Solid Edge part; units mm, degrees
sketch "Sketch1" plane through (0, 0, 0) normal (0, -1, 0) x (1, 0, 0)
  circle A0 centre (0, 0) radius 6
extrude "Protrusion1" add sketch "Sketch1" along normal blind 3.6
sketch "Sketch2" plane through (0, -3.6, 0) normal (0, -1, 0) x (1, 0, 0)
  circle A0 centre (0, 0) radius 3
extrude "Protrusion2" add sketch "Sketch2" along normal blind 20
sketch "Sketch3" plane through (0, 0, 0) normal (0, 1, 0) x (0, 0, -1)
  line L0 (2.5, -1.4434) -> (2.5, 1.4434)
  line L1 (2.5, 1.4434) -> (0, 2.8868)
  line L2 (0, 2.8868) -> (-2.5, 1.4434)
  line L3 (-2.5, 1.4434) -> (-2.5, -1.4434)
  line L4 (-2.5, -1.4434) -> (0, -2.8868)
  line L5 (0, -2.8868) -> (2.5, -1.4434)
extrude "ExtrudedCutout_4" cut sketch "Sketch3" against normal blind 3
properties material "Nylon, general purpose"
Read the model definition and answer for the solid it produces. Units are mm, in the model's axes. A direction names the side the tool comes from. Round coordinates to 2 decimals unless told otherwise and drop trailing zeros. Write each loop counter-clockwise with the first axis right and the second up, starting at its lowest first coordinate (ties: lowest second). Pieces come first, ordered by that corner, then holes. Notation, with made-up numbers: M 57,-17.75 L 79,-17.75 A20 ccw 79,-3.75 Z; hole C -20,15 d3. An arc over 180 degrees is marked long. One line per item, written item: value.
Q1. Straight lines are drawn through the part: line 1 (Y direction, x = 4, z = 3.75); line 2 (Y direction, x = 0, z = -2.25); line 3 (Z direction, x = -1, y = -1). For each, find the intervals that lie inside material, in ascending order. Write a range as [from, to].
Data:
line 1: [-3.6, 0]
line 2: [-23.6, -3]
line 3: [-5.92, -2.5], [2.5, 5.92]
Q2. Which of the six approach directions +Z, -Z, +X, -X, +Y, -Y give full straight-line access (tool end or side, diameter ignored) to faces 5 (the flat face through (-1, -3.6, 3)), 6 (the flat face through (-2.175, -1.479, 1.233)), 7 (the flat face through (0, -23.6, 0))?
Data:
face 5: -Y
face 6: +Y
face 7: +Z, -Z, +X, -X, -Y
Q3. Find section D-D on x = -3.5. Write down the section's boundary in (y, z).
Data:
outline: M -3.6,-4.87 L 0,-4.87 L 0,4.87 L -3.6,4.87 Z
Q4. For a pull along Z with two mould halves and no side action, classify faces 1 (the flat face through (0, 0, -3)), 2 (the flat face through (0, -1, -2.5)), 3 (the cylindrical face through (-3, -13, 0)), 4 (the flat face through (2.155, -1.479, 1.267)) as +Z half, -Z half, draft (parallel to the pull), parting line (faces both ways), or undercut.
Data:
face 1: draft
face 2: undercut
face 3: parting line
face 4: undercut
Q5. Flat-ended cylindrical pins translate along their axes: pin 1 Ø5 at (x, y) = (3, -18.5) entering from -Z; pin 2 Ø2 at (y, z) = (-10, 0.5) entering from +X; pin 3 Ø6 at (y, z) = (-18, -4.5) entering from +X. Find the tip coordinate at first contact, or state that the pin passes through.
Data:
pin 1: z = -2.96
pin 2: x = 3
pin 3: x = 2.6
Q6. Find section A-A on x = 0. Write down the section's boundary in (y, z), plus the area to 3 significant figures.
Data:
outline: M -23.6,-3 L -3.6,-3 L -3.6,-6 L 0,-6 L 0,-2.5 L -3,-2.5 L -3,2.5 L 0,2.5 L 0,6 L -3.6,6 L -3.6,3 L -23.6,3 Z
area: 148 mm2
Q7. Find section B-B on z = 2. Write down the section's boundary in (x, y).
Data:
outline: M -5.66,-3.6 L -2.24,-3.6 L -2.24,-23.6 L 2.24,-23.6 L 2.24,-3.6 L 5.66,-3.6 L 5.66,0 L 1.73,0 L 1.73,-3 L -1.73,-3 L -1.73,0 L -5.66,0 Z
Q8. Find section C-C on y = -6.75. Write down the section's boundary in (x, z), plus the area to 3 significant figures.
Data:
outline: C 0,0 d6
area: 28.3 mm2
